```python
from build123d import *

# Parameters (mm, degrees)
F1_DEPTH  = 30
F2_R      = 4.5
F2_R_2    = 2.75
F3_DEPTH  = 5
F3_FACE_R = 2.75
F4_DEPTH  = 12
F5_R      = 1


with BuildPart() as f1:
    # F0 (on Top) → F1 (new body)
    with BuildSketch(Plane.XY):
        with BuildLine():
            ThreePointArc((-12.031281, -1), (-14.000959, -7.7477), (-18.672621, -13))
            Line((-18.672621, -13), (18.672621, -13))
            ThreePointArc((18.672621, -13), (14.000959, -7.7477), (12.031281, -1))
            Line((12.031281, -1), (-12.031281, -1))
        make_face()
    extrude(amount=F1_DEPTH)

    # F2 (on face) → F3 (cut)
    with BuildSketch(Plane.XZ.offset(13)):
        with Locations((0, 15)):
            Circle(F2_R)
        with Locations((0, 15)):
            Circle(F2_R_2, mode=Mode.SUBTRACT)
    extrude(amount=-F3_DEPTH, mode=Mode.SUBTRACT)

    # F3_face (on face) → F4 (cut, through all)
    with BuildSketch(Plane(origin=(0, -13, 15), x_dir=(1, 0, 0), z_dir=(0, -1, 0))):
        Circle(F3_FACE_R)
    extrude(amount=-F4_DEPTH, mode=Mode.SUBTRACT)

    # F5
    f5_edges = [f1.edges().sort_by_distance(p)[0] for p in [
        (-18.672621, -13, 15),
        (-12.031281, -1, 15),
        (18.672621, -13, 15),
        (12.031281, -1, 15),
    ]]
    fillet(f5_edges, radius=F5_R)


solid = f1.part
```
Read the model definition and answer for the solid it produces. Units are mm, in the model's axes. A direction names the side the tool comes from. Give positions to 0.01 mm unless a question says otherwise; leave off trailing zeros. Order: outer loops, then holes, each group sorted by start corner. A loop starts at its lowest first (then second) coordinate and runs counter-clockwise, first axis right, second up. Notation, with made-up numbers: (20, 1.5) -> (49, 1.5) arc R10 cw to (49, 8.5) -> close; hole circle Ø10 at (-1, 1). An arc over 180 degrees is marked (long way). One line per item, written item: value. Start each with the question number.
(1) The part is cut by section A-A (z = 15). Determine the outline of the cut face in (x, y), and give its area (3 significant figures).
(2) For a pull along Z with two mould halves and no side action, classify faces 3 (the cylindrical face through (-0.358, -4.549, 17.727)), 4 (the flat face through (0, -7, 0)), 5 (the cylindrical face through (-11.79, -1.26, 15.21)) as released by +Z, released by -Z, zero draft, split by the parting line, or undercut.
(3) The part is cut by section D-D (z = 2.5). Determine the outline of the cut face in (x, y), and give its area (3 significant figures).
(4) The part is cut by section C-C (y = -10). Determine the outline of the cut face in (x, z), and give its area (3 significant figures).
(5) The part is cut by section B-B (x = 0). Determine the outline of the cut face in (y, z).
(6) A tool of negligible diameter and unlimited length cuts with its end or side. For faces 1 (the flat face through (0, -8, 12)), 2 (the flat face through (0, -7, 30)), from which of +Z, -Z, +X, -X, +Y, -Y can it reach the whole face along a straight path? Write none if from no direction.
(7) Straight lines are drawn through the part: L1, parallel to Z at x = 0, y = -2.25; L2, parallel to Z at x = 0, y = -11.3; L3, parallel to X at y = -6.25, z = 25.25. For each, find the intervals that lie inside material, in ascending order.
(8) Flat-ended cylindrical pins translate along their axes: P1, Ø4.5, axis at x = 0, z = 15, coming from the -Y side; P2, Ø4, axis at y = -6.5, z = 4.5, coming from the -X side. Find the tip coordinate at first contact, or state that the pin passes through.
Taken from the geometry:
1. outline: (-16.67, -11.29) arc R1 ccw to (-15.96, -13) -> (-4.5, -13) -> (-4.5, -8) -> (-2.75, -8) -> (-2.75, -1) -> (-11.12, -1) arc R1 ccw to (-12.11, -1.88) arc R16 cw to start; (2.75, -8) -> (4.5, -8) -> (4.5, -13) -> (15.96, -13) arc R1 ccw to (16.67, -11.29) arc R16 cw to (12.11, -1.88) arc R1 ccw to (11.12, -1) -> (2.75, -1) -> close
1. area: 253 mm^2
2. face 3: undercut
2. face 4: released by -Z
2. face 5: zero draft
3. outline: (-16.67, -11.29) arc R1 ccw to (-15.96, -13) -> (15.96, -13) arc R1 ccw to (16.67, -11.29) arc R16 cw to (12.11, -1.88) arc R1 ccw to (11.12, -1) -> (-11.12, -1) arc R1 ccw to (-12.11, -1.88) arc R16 cw to start
3. area: 337 mm^2
4. outline: (-15.51, 0) -> (15.51, 0) -> (15.51, 30) -> (-15.51, 30) -> close; hole circle Ø9 at (0, 15)
4. area: 867 mm^2
5. outline: (-13, 0) -> (-1, 0) -> (-1, 12.25) -> (-8, 12.25) -> (-8, 10.5) -> (-13, 10.5) -> close; (-13, 19.5) -> (-8, 19.5) -> (-8, 17.75) -> (-1, 17.75) -> (-1, 30) -> (-13, 30) -> close
6. face 1: -Y
6. face 2: +Z, +X, -X, +Y, -Y
7. L1: 0 to 12.25, 17.75 to 30
7. L2: 0 to 10.5, 19.5 to 30
7. L3: -13.27 to 13.27
8. P1: through
8. P2: x = -14.44
